```python
from build123d import *

# Parameters (mm, degrees)
F0_R     = 38.1
F1_DEPTH = 123.825
F2_R     = 34.925
F3_DEPTH = 111.125
F5_R     = 7.62


# Not quite as in the source:
# - a fillet or chamfer that OpenCascade refuses, or shapes differently, is made with other operations: its cross-section is extruded or revolved along the edge and cut away or added


with BuildPart() as f1:
    # F0 (on Top) → F1 (new body)
    with BuildSketch(Plane.XY):
        Circle(F0_R)
    extrude(amount=F1_DEPTH)

    # F2 (on Top) → F3 (cut)
    with BuildSketch(Plane.XY):
        Circle(F2_R)
    extrude(amount=F3_DEPTH, mode=Mode.SUBTRACT)

    # F4: fillet of radius 7.62 on 1 edges, made by hand

    # F4_s1 → F4_t2 (revolve, cut)
    with BuildSketch(Plane.XZ):
        with BuildLine():
            ThreePointArc((38.1, 6.189214409), (37.25994469, 2.7111761688), (34.925, 0))
            Line((34.925, 0), (38.1, 0))
            Line((38.1, 0), (38.1, 6.189214409))
        make_face()
    revolve(axis=Axis((0, 0, 0), (0, 0, 1)), mode=Mode.SUBTRACT)

    # F5
    f5_edges = [f1.edges().sort_by_distance(p)[0] for p in [
        (-38.1, 0, 123.825),
    ]]
    fillet(f5_edges, radius=F5_R)


solid = f1.part
```
The model under review builds one solid part; all positions refer to its coordinate system, in mm. Coordinates: 2 decimals unless noted, no trailing zeros. Write each loop counter-clockwise with the first axis right and the second up, starting at its lowest first coordinate (ties: lowest second). Pieces come first, ordered by that corner, then holes.
1) We need section C-C on z = 92. State the section outline as (x, y) points (3 decimals), then the cut area to 3 significant figures.
2) The part is to be moulded in two halves that separate along X. For faces 1 (the face through (0, 0, 111.125)), 2 (the face through (-30.235, -23.183, 60.427)), 3 (the face through (0, 0, 123.825)), say which applies: pulls with the +X half, pulls with the -X half, needs draft (parallel to the pull), parting line crosses it, or undercut.
3) To check wall thickness, follow probe 1 along Y at (x, z) = (0, 35.5) (3 decimals); probe 2 along Y at (x, z) = (-17, 11); probe 3 along X at (y, z) = (-6.5, 41.5). State the ranges of each line that lie inside material, in increasing order.
4) We need section A-A on y = 0. State the section outline as (x, z) points (3 decimals).
5) Clearance check with flat-ended pins moving along their axes: pin 1 Ø8 at (x, z) = (-18, 67.5) entering from -Y; pin 2 Ø1.5 at (x, z) = (24.5, 67.5) entering from -Y; pin 3 Ø6 at (x, y) = (24, 26) entering from +Z. State where each tip first meets the part, or that it passes through.
Answer list:
1. outline: circle Ø76.2 at (0, 0); hole circle Ø69.85 at (0, 0)
1. area: 728 mm2
2. face 1: undercut
2. face 2: parting line crosses it
2. face 3: needs draft
3. probe 1: y = -38.1 to -34.925, 34.925 to 38.1
3. probe 2: y = -34.1 to -30.51, 30.51 to 34.1
3. probe 3: x = -37.54 to -34.31, 34.31 to 37.54
4. outline: (-38.1, 6.189) arc R7.62 ccw to (-34.925, 0) - (-34.925, 111.125) - (34.925, 111.125) - (34.925, 0) arc R7.62 ccw to (38.1, 6.189) - (38.1, 116.205) arc R7.62 ccw to (30.48, 123.825) - (-30.48, 123.825) arc R7.62 ccw to (-38.1, 116.205) - close
5. pin 1: stops at y = -35.43
5. pin 2: stops at y = -29.79
5. pin 3: stops at z = 123.58
